The figure shows three views and two pictorial views of one solid part (mm, origin at its lowest corner). Answer the questions. A direction names the side the tool comes from. Give positions to 0.01 mm unless a question says otherwise; leave off trailing zeros. Loops run counter-clockwise (first coordinate to the right, second up) from the corner with the lowest first, then second, coordinate; pieces in that order, holes last. Notation, with made-up numbers: (59, 27) - (104, 27) arc R21 ccw to (104, 65) - close; hole circle Ø8 at (65, 23.5). An arc over 180 degrees is marked (long way). Write each question's results on one line, items separated by ' | '.
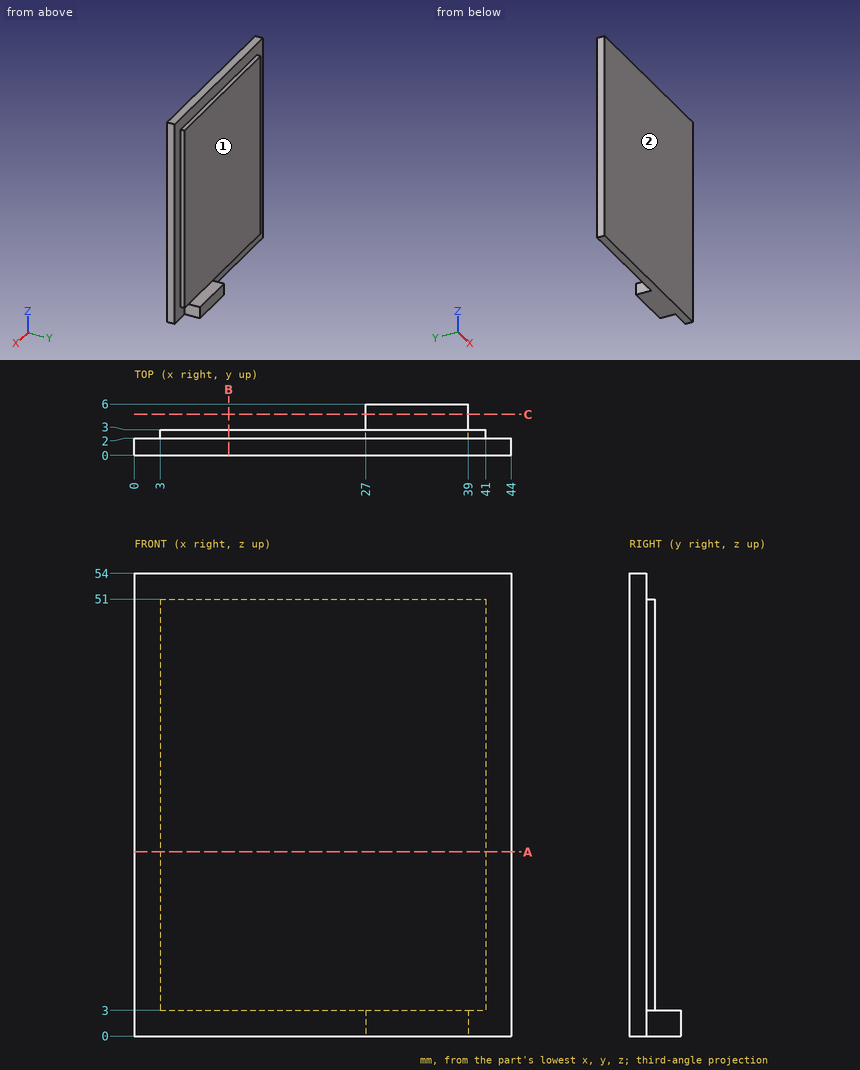
Item 1: For the marked faces 1 and 2, determine the directions among +Z, -Z, +X, -X, +Y, -Y from which every point of the face is accessible in a straight line to the end or side of a thin tool.
Values found:
face 1: +Z, +X, -X, +Y | face 2: +Z, -Z, +X, -X, -Y
Item 2: A cutting plane is placed at C-C, the plane y = 4.8. Determine the outline of the cut face in (x, z), plus the area to 3 significant figures.
Values found:
outline: (27, 0) - (39, 0) - (39, 3) - (27, 3) - close | area: 36.0 mm²
Item 3: A cutting plane is placed at B-B, the plane x = 11. Determine the outline of the cut face in (y, z).
Values found:
outline: (0, 0) - (2, 0) - (2, 3) - (3, 3) - (3, 51) - (2, 51) - (2, 54) - (0, 54) - close
Item 4: Flat-ended cylindrical pins translate along their axes: P1, Ø5, axis at x = 29, z = 32.5, coming from the +Y side; P2, Ø0.8, axis at y = 2.5, z = 31, coming from the +X side; P3, Ø0.8, axis at x = 15.5, y = 2.5, coming from the -Z side. Find the tip coordinate at first contact, or state that the pin passes through.
Values found:
P1: stops at y = 3 | P2: stops at x = 41 | P3: stops at z = 3
Item 5: Find the intervals of material crossed by line 1 along Y through (x, z) = (28, 12); line 2 along Z through (x, y) = (4, 2.5), in increasing order. Write a range as [from, to].
Values found:
line 1: y = [0, 3] | line 2: z = [3, 51]
Item 6: A cutting plane is placed at A-A, the plane z = 21.5. Determine the outline of the cut face in (x, y).
Values found:
outline: (0, 0) - (44, 0) - (44, 2) - (41, 2) - (41, 3) - (3, 3) - (3, 2) - (0, 2) - close
